Design review of the part shown in the three views and the two pictorial views. Dimensions are in mm from the part's minimum x, y and z. A direction names the side the tool comes from. Give positions to 0.01 mm unless a question says otherwise; leave off trailing zeros. Loops run counter-clockwise (first coordinate to the right, second up) from the corner with the lowest first, then second, coordinate; pieces in that order, holes last.
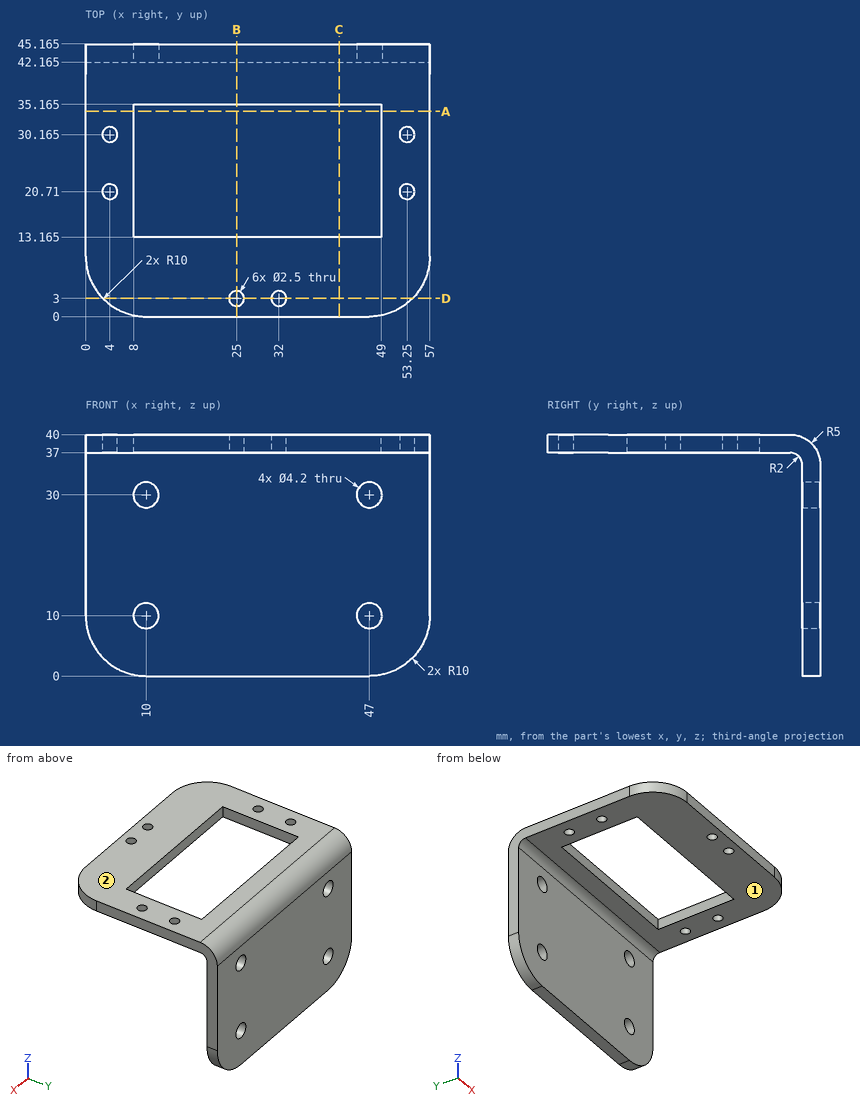
Q1. Take a section at A-A (y = 34). Give the boundary of the cut face in (x, z).
Results:
outline: (0, 37) - (8, 37) - (8, 40) - (0, 40) - close; (49, 37) - (57, 37) - (57, 40) - (49, 40) - close
Q2. Wall thickness on line 1 (Y direction, x = 4, z = 38.25) (1 decimal); line 2 (Y direction, x = 39.5, z = 6) (1 decimal); line 3 (Z direction, x = 11, y = 38): over which ranges is each line inside the solid? List them lowest first.
Results:
line 1: y = 2 to 19.5, 22 to 28.9, 31.4 to 44
line 2: y = 42.2 to 45.2
line 3: z = 37 to 40
Q3. Take a section at D-D (y = 3). Give the boundary of the cut face in (x, z), plus the area to 3 significant figures.
Results:
outline: (2.86, 37) - (23.75, 37) - (23.75, 40) - (2.86, 40) - close; (26.25, 37) - (30.75, 37) - (30.75, 40) - (26.25, 40) - close; (33.25, 37) - (54.14, 37) - (54.14, 40) - (33.25, 40) - close
area: 139 mm2
Q4. Tool access review of the marked faces 1 and 2: name each direction out of +Z, -Z, +X, -X, +Y, -Y from which nothing blocks a thin tool from reaching the whole face with its end or side.
Results:
face 1: -Z, +X, -X, -Y
face 2: +Z, +X, -X, +Y, -Y
Q5. Take a section at B-B (x = 25). Give the number of separate pieces and of enclosed holes in the cut face.
Results:
separate pieces: 3
enclosed holes: 0
Q6. Insertion check: pin 1 (2.5 mm diameter, centred on x = 47, z = 10, fed in from +Y); pin 2 (5 mm diameter, centred on x = 10, z = 10, fed in from -Y) (1 decimal); pin 3 (1.5 mm diameter, centred on x = 28.5, z = 39, fed in from +Y) (1 decimal); pin 4 (2.5 mm diameter, centred on x = 29.5, z = 39, fed in from -Y). Each pin has a flat end and moves straight along its axis. Give the tip position at first contact, or say it passes through.
Results:
pin 1: passes through
pin 2: stops at y = 42.2
pin 3: stops at y = 44
pin 4: stops at y = 0
Q7. Take a section at C-C (x = 42). Give the boundary of the cut face in (y, z) (1 decimal), plus the area to 3 significant figures.
Results:
outline: (0, 37) - (13.2, 37) - (13.2, 40) - (0, 40) - close; (35.2, 37) - (40.2, 37) arc R2 cw to (42.2, 35) - (42.2, 0) - (45.2, 0) - (45.2, 35) arc R5 ccw to (40.2, 40) - (35.2, 40) - close
area: 176 mm2
